```python
from build123d import *

# Parameters (mm, degrees)
EXTRUDE_1_OUTLINE_W    = 15
EXTRUDE_1_OUTLINE_H    = 15
EXTRUDE_1_DEPTH        = 8
SKETCH_2_W             = 6
SKETCH_2_H             = 11
CUT_EXTRUDE_1_DEPTH    = 13
SKETCH_3_W             = 3
SKETCH_3_H             = 15
EXTRUDE_2_DEPTH        = 2
PATTERN_LINEAR_2_COUNT = 11
PATTERN_LINEAR_2_PITCH = 10
SKETCH_5_W             = 12
SKETCH_5_H             = 15
EXTRUDE_3_DEPTH        = 2
SKETCH_6_W             = 15
SKETCH_6_H             = 15
EXTRUDE_4_DEPTH        = 2
SKETCH_7_W             = 94
SKETCH_7_H             = 2
CUT_EXTRUDE_2_DEPTH    = 2
SKETCH_9_W             = 108
SKETCH_9_H             = 13
SKETCH_9_W_2           = 106
SKETCH_9_H_2           = 11
EXTRUDE_5_DEPTH        = 2
SKETCH_10_W            = 2
SKETCH_10_H            = 2.5
EXTRUDE_6_DEPTH        = 2


# Read off the part's stored shape, not the designer's step: 凸台-拉伸1
with BuildPart() as part:
    # 凸台-拉伸1 outline → 凸台-拉伸1 (new body)
    with BuildSketch(Plane.YZ):
        with Locations((7.5, -7.5)):
            Rectangle(EXTRUDE_1_OUTLINE_W, EXTRUDE_1_OUTLINE_H)
    extrude(amount=EXTRUDE_1_DEPTH)

    # 草图2 → 切除-拉伸1 (cut)
    with BuildSketch(Plane.XY):
        with Locations((4, 7.5)):
            Rectangle(SKETCH_2_W, SKETCH_2_H)
    extrude(amount=-CUT_EXTRUDE_1_DEPTH, mode=Mode.SUBTRACT)

    # 草图3 → 凸台-拉伸2 (add)
    with BuildSketch(Plane(origin=(8, 0, 0), x_dir=(0, 0, -1), z_dir=(1, 0, 0))):
        with Locations((1.5, 7.5)):
            Rectangle(SKETCH_3_W, SKETCH_3_H)
    extrude(amount=EXTRUDE_2_DEPTH)


with BuildPart() as pattern_linear_2_1:
    # 阵列(线性)2: pattern copy
    add(part.part.moved(Location(Vector(1, 0, 0) * (1 * PATTERN_LINEAR_2_PITCH))))


with BuildPart() as pattern_linear_2_2:
    # 阵列(线性)2: pattern copy
    add(part.part.moved(Location(Vector(1, 0, 0) * (2 * PATTERN_LINEAR_2_PITCH))))


with BuildPart() as pattern_linear_2_3:
    # 阵列(线性)2: pattern copy
    add(part.part.moved(Location(Vector(1, 0, 0) * (3 * PATTERN_LINEAR_2_PITCH))))


with BuildPart() as pattern_linear_2_4:
    # 阵列(线性)2: pattern copy
    add(part.part.moved(Location(Vector(1, 0, 0) * (4 * PATTERN_LINEAR_2_PITCH))))


with BuildPart() as pattern_linear_2_5:
    # 阵列(线性)2: pattern copy
    add(part.part.moved(Location(Vector(1, 0, 0) * (5 * PATTERN_LINEAR_2_PITCH))))


with BuildPart() as pattern_linear_2_6:
    # 阵列(线性)2: pattern copy
    add(part.part.moved(Location(Vector(1, 0, 0) * (6 * PATTERN_LINEAR_2_PITCH))))


with BuildPart() as pattern_linear_2_7:
    # 阵列(线性)2: pattern copy
    add(part.part.moved(Location(Vector(1, 0, 0) * (7 * PATTERN_LINEAR_2_PITCH))))


with BuildPart() as pattern_linear_2_8:
    # 阵列(线性)2: pattern copy
    add(part.part.moved(Location(Vector(1, 0, 0) * (8 * PATTERN_LINEAR_2_PITCH))))


with BuildPart() as pattern_linear_2_9:
    # 阵列(线性)2: pattern copy
    add(part.part.moved(Location(Vector(1, 0, 0) * (9 * PATTERN_LINEAR_2_PITCH))))


with BuildPart() as pattern_linear_2_10:
    # 阵列(线性)2: pattern copy
    add(part.part.moved(Location(Vector(1, 0, 0) * (10 * PATTERN_LINEAR_2_PITCH))))


with BuildPart() as part_1:
    add(part.part)

    # Combine 2: union 阵列(线性)2_1, 阵列(线性)2_2, 阵列(线性)2_3, 阵列(线性)2_4, 阵列(线性)2_5, 阵列(线性)2_6, 阵列(线性)2_7, 阵列(线性)2_8, 阵列(线性)2_9, 阵列(线性)2_10
    add(pattern_linear_2_1.part)
    add(pattern_linear_2_2.part)
    add(pattern_linear_2_3.part)
    add(pattern_linear_2_4.part)
    add(pattern_linear_2_5.part)
    add(pattern_linear_2_6.part)
    add(pattern_linear_2_7.part)
    add(pattern_linear_2_8.part)
    add(pattern_linear_2_9.part)
    add(pattern_linear_2_10.part)

    # 草图5 → 凸台-拉伸3 (add)
    with BuildSketch(Plane(origin=(108, 0, 0), x_dir=(0, 0, -1), z_dir=(1, 0, 0))):
        with Locations((9, 7.5)):
            Rectangle(SKETCH_5_W, SKETCH_5_H)
    extrude(amount=EXTRUDE_3_DEPTH)

    # 草图6 → 凸台-拉伸4 (add)
    with BuildSketch(Plane.ZY):
        with Locations((-7.5, 7.5)):
            Rectangle(SKETCH_6_W, SKETCH_6_H)
    extrude(amount=EXTRUDE_4_DEPTH)

    # 草图7 → 切除-拉伸2 (cut)
    with BuildSketch(Plane.XY):
        with Locations((54, 7.5)):
            Rectangle(SKETCH_7_W, SKETCH_7_H)
    extrude(amount=-CUT_EXTRUDE_2_DEPTH, mode=Mode.SUBTRACT)

    # 草图9 → 凸台-拉伸5 (add)
    with BuildSketch(Plane.XY):
        with Locations((54, 7.5)):
            Rectangle(SKETCH_9_W, SKETCH_9_H)
        with Locations((54, 7.5)):
            Rectangle(SKETCH_9_W_2, SKETCH_9_H_2, mode=Mode.SUBTRACT)
    extrude(amount=EXTRUDE_5_DEPTH)

    # 草图10 → 凸台-拉伸6 (add)
    with BuildSketch(Plane.XY):
        with Locations((9, 4.25)):
            Rectangle(SKETCH_10_W, SKETCH_10_H)
        with Locations((9, 10.75)):
            Rectangle(SKETCH_10_W, SKETCH_10_H)
    extrude(amount=EXTRUDE_6_DEPTH)


solid = part_1.part
```
Model file for the job. Use its own axes, mm. A direction names the side the tool comes from. Give positions to 0.01 mm unless a question says otherwise; leave off trailing zeros. Write each loop counter-clockwise with the first axis right and the second up, starting at its lowest first coordinate (ties: lowest second). Pieces come first, ordered by that corner, then holes. Notation, with made-up numbers: (66.25, -18.5) - (116.25, -18.5) arc R17 ccw to (116.25, 0.5) - close; hole circle Ø2 at (83.5, -28.75). An arc over 180 degrees is marked (long way). One line per question, with ' | ' between items. Start each with the question number.
(1) Wall check: line 1 along Y through (x, z) = (61.5, -1.5); line 2 along Y through (x, z) = (48, 1); line 3 along Z through (x, y) = (56, 3.75). Give the ranges that are in metal, low to high. Write a range as from..to.
(2) Slice it at D-D on x = 99. Write the cut outline in (y, z), plus the area to 3 significant figures.
(3) Pin check, flat tips, straight feed: P1, Ø2, axis at x = 78.5, y = 8, coming from the +Z side; P2, Ø1.6, axis at y = 10.5, z = 1, coming from the -X side; P3, Ø0.6, axis at x = 38.5, y = 7.5, coming from the +Z side. Stop position of each tip, or through.
(4) Slice it at A-A on x = 9. Write the cut outline in (y, z).
(5) Slice it at B-B on z = -6. Give the number of separate pieces and of enclosed holes in the cut face, plus the area to 3 significant figures.
(6) Slice it at C-C on x = 54. Write the cut outline in (y, z).
(7) 3-axis set-ups, long thin cutter, end or side, ignore diameter. For faces 3 (the face through (9, 12, 1)), 4 (the face through (64, 7, -15)), 5 (the face through (69, 7, -3)): which of +Z, -Z, +X, -X, +Y, -Y reach the whole face in a straight line?
(8) Two-plate mould, pull along X, no slides. Class faces 1 (the face through (39, 11, 0)), 2 (the face through (84, 7, -15)): +X half, -X half, draft (parallel to the pull), parting line (faces both ways), or undercut.
Results below:
1) line 1: 0..2, 13..15 | line 2: 1..2, 13..14 | line 3: -15..-13
2) outline: (0, -3) - (15, -3) - (15, 0) - (14, 0) - (14, 2) - (13, 2) - (13, 0) - (8.5, 0) - (8.5, -2) - (6.5, -2) - (6.5, 0) - (2, 0) - (2, 2) - (1, 2) - (1, 0) - (0, 0) - close | area: 45.0 mm^2
3) P1: z = 0 | P2: x = 0 | P3: z = -2
4) outline: (0, -3) - (15, -3) - (15, 0) - (14, 0) - (14, 2) - (13, 2) - (13, 0) - (12, 0) - (12, 2) - (9.5, 2) - (9.5, 0) - (8.5, 0) - (8.5, -2) - (6.5, -2) - (6.5, 0) - (5.5, 0) - (5.5, 2) - (3, 2) - (3, 0) - (2, 0) - (2, 2) - (1, 2) - (1, 0) - (0, 0) - close
5) separate pieces: 11 | enclosed holes: 11 | area: 654 mm^2
6) outline: (0, -15) - (15, -15) - (15, 0) - (14, 0) - (14, 2) - (13, 2) - (13, -13) - (2, -13) - (2, 2) - (1, 2) - (1, 0) - (0, 0) - close
7) face 3: +Z | face 4: -Z, +X, -X, +Y, -Y | face 5: -Z, +Y, -Y
8) face 1: undercut | face 2: draft
